```python
from build123d import *

# Parameters (mm, degrees)
SKETCH1_R               = 7.5
BOSS_EXTRUDE1_DEPTH     = 10
SKETCH2_R               = 15
BOSS_EXTRUDE2_DEPTH     = 5
SKETCH3_R               = 6
BOSS_EXTRUDE3_DEPTH     = 40
SKETCH4_R               = 15
BOSS_EXTRUDE4_DEPTH     = 5
SKETCH5_R               = 7.5
BOSS_EXTRUDE5_DEPTH     = 10
CUT_EXTRUDE1_DEPTH      = 74.143694192
CUT_EXTRUDE1_DEPTH_BACK = 74.143694192
SKETCH6_R               = 1


with BuildPart() as part:
    # Sketch1 → Boss-Extrude1 (new body)
    with BuildSketch(Plane(origin=(0, 0, 0), x_dir=(1, 0, 0), z_dir=(0, 1, 0))):
        with Locations(Location((0, 0, 0), (0, 0, 270))):
            Circle(SKETCH1_R)
    extrude(amount=BOSS_EXTRUDE1_DEPTH)

    # Sketch2 → Boss-Extrude2 (add)
    with BuildSketch(Plane(origin=(0, 10, 0), x_dir=(1, 0, 0), z_dir=(0, 1, 0))):
        with Locations(Location((0, 0, 0), (0, 0, 270))):
            Circle(SKETCH2_R)
    extrude(amount=BOSS_EXTRUDE2_DEPTH)

    # Sketch3 → Boss-Extrude3 (add)
    with BuildSketch(Plane(origin=(0, 15, 0), x_dir=(1, 0, 0), z_dir=(0, 1, 0))):
        with Locations(Location((0, 0, 0), (0, 0, 270))):
            Circle(SKETCH3_R)
    extrude(amount=BOSS_EXTRUDE3_DEPTH)

    # Sketch4 → Boss-Extrude4 (add)
    with BuildSketch(Plane(origin=(0, 55, 0), x_dir=(1, 0, 0), z_dir=(0, 1, 0))):
        with Locations(Location((0, 0, 0), (0, 0, 270))):
            Circle(SKETCH4_R)
    extrude(amount=BOSS_EXTRUDE4_DEPTH)

    # Sketch5 → Boss-Extrude5 (add)
    with BuildSketch(Plane(origin=(0, 60, 0), x_dir=(1, 0, 0), z_dir=(0, 1, 0))):
        with Locations(Location((0, 0, 0), (0, 0, 270))):
            Circle(SKETCH5_R)
    extrude(amount=BOSS_EXTRUDE5_DEPTH)

    # Sketch6 → Cut-Extrude1 (cut, two sides: drawn at the far end of the back side and taken through both)
    with BuildSketch(Plane.XY.offset(-CUT_EXTRUDE1_DEPTH_BACK)):
        with Locations((0, 4)):
            Circle(SKETCH6_R)
        with Locations((0, 66)):
            Circle(SKETCH6_R)
    extrude(amount=CUT_EXTRUDE1_DEPTH + CUT_EXTRUDE1_DEPTH_BACK, mode=Mode.SUBTRACT)


solid = part.part
```
Work out the finished part from the listing and answer in its coordinate system (mm). A direction names the side the tool comes from. Coordinates: 2 decimals unless noted, no trailing zeros. Loops run counter-clockwise (first coordinate to the right, second up) from the corner with the lowest first, then second, coordinate; pieces in that order, holes last. Notation, with made-up numbers: (-5, 33.5) -> (51, 33.5) arc R23 cw to (51, 57.5) -> close; hole circle Ø8 at (-10.75, -25.75). An arc over 180 degrees is marked (long way). Answer as CSV lines item,"result".
Q1. The part is cut by section C-C on z = -9.5. Write down the section's boundary in (x, y).
Findings:
outline,"(-11.61, 10) -> (11.61, 10) -> (11.61, 15) -> (-11.61, 15) -> close; (-11.61, 55) -> (11.61, 55) -> (11.61, 60) -> (-11.61, 60) -> close"
Q2. A tool of negligible diameter and unlimited length cuts with its end or side. For faces 1 (the face through (7, 60, -4)), 2 (the face through (0.2, 55, 6.5)), 3 (the face through (-2.87, 4.93, 6.93)), from which of +Z, -Z, +X, -X, +Y, -Y can it reach the whole face along a straight path? Write none if from no direction.
Findings:
face 1,"+Y"
face 2,"none"
face 3,"-Y"
Q3. The part is cut by section B-B on x = 0. Write down the section's boundary in (y, z), and give its area (3 significant figures).
Findings:
outline,"(0, -7.5) -> (3, -7.5) -> (3, 7.5) -> (0, 7.5) -> close; (5, -7.5) -> (10, -7.5) -> (10, -15) -> (15, -15) -> (15, -6) -> (55, -6) -> (55, -15) -> (60, -15) -> (60, -7.5) -> (65, -7.5) -> (65, 7.5) -> (60, 7.5) -> (60, 15) -> (55, 15) -> (55, 6) -> (15, 6) -> (15, 15) -> (10, 15) -> (10, 7.5) -> (5, 7.5) -> close; (67, -7.5) -> (70, -7.5) -> (70, 7.5) -> (67, 7.5) -> close"
area,"1,020 mm²"
Q4. The part is cut by section D-D on z = 0. Write down the section's boundary in (x, y), and give its area (3 significant figures).
Findings:
outline,"(-15, 10) -> (-7.5, 10) -> (-7.5, 0) -> (7.5, 0) -> (7.5, 10) -> (15, 10) -> (15, 15) -> (6, 15) -> (6, 55) -> (15, 55) -> (15, 60) -> (7.5, 60) -> (7.5, 70) -> (-7.5, 70) -> (-7.5, 60) -> (-15, 60) -> (-15, 55) -> (-6, 55) -> (-6, 15) -> (-15, 15) -> close; hole circle Ø2 at (0, 4); hole circle Ø2 at (0, 66)"
area,"1,070 mm²"
Q5. Each of these flat-tipped pins is pushed along its axis until it touches: pin 1 (2.5 mm diameter, centred on x = 0, y = 66, fed in from +Z); pin 2 (6 mm diameter, centred on x = -8.5, z = 10.5, fed in from -Y); pin 3 (10 mm diameter, centred on x = 1, y = 43, fed in from -Z); pin 4 (1.2 mm diameter, centred on x = 0, y = 4, fed in from -Z). Where does it stop, or does it pass through?
Findings:
pin 1,"stops at z = 7.5"
pin 2,"stops at y = 10"
pin 3,"stops at z = -6"
pin 4,"passes through"
Q6. The part is cut by section A-A on x = -12. Write down the section's boundary in (y, z).
Findings:
outline,"(10, -9) -> (15, -9) -> (15, 9) -> (10, 9) -> close; (55, -9) -> (60, -9) -> (60, 9) -> (55, 9) -> close"
Q7. For a pull along Y with two mould halves and no side action, classify faces 4 (the face through (0.66, 12.465, -14.985)), 5 (the face through (0, 70, 0)), 6 (the face through (0.2, 15, 6.5)) as +Y half, -Y half, draft (parallel to the pull), parting line (faces both ways), or undercut.
Findings:
face 4,"draft"
face 5,"+Y half"
face 6,"undercut"
Q8. Find the intervals of material crossed by probe 1 along Y at (x, z) = (0, -3); probe 2 along X at (y, z) = (4, 0.5); probe 3 along Y at (x, z) = (-12, -7.25), in increasing order.
Findings:
probe 1,"y = 0 to 3, 5 to 65, 67 to 70"
probe 2,"x = -7.48 to -1, 1 to 7.48"
probe 3,"y = 10 to 15, 55 to 60"
